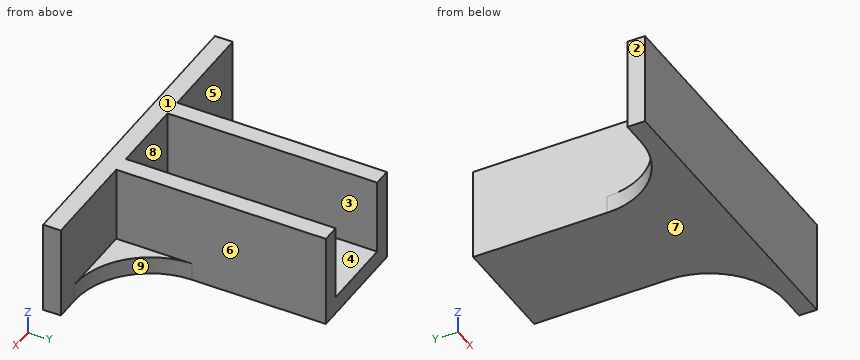
```python
from build123d import *

# Parameters (mm, degrees)
SKETCH1_W           = 22
SKETCH1_H           = 45
BOSS_EXTRUDE1_DEPTH = 18.5
SKETCH2_W           = 15
SKETCH2_H           = 41.5
CUT_EXTRUDE1_DEPTH  = 15
SKETCH3_W           = 20
SKETCH3_H           = 3.5
BOSS_EXTRUDE2_DEPTH = 18.5
BOSS_EXTRUDE3_DEPTH = 3.5


with BuildPart() as part:
    # Sketch1 → Boss-Extrude1 (new body)
    with BuildSketch(Plane.XY):
        with Locations((-5.139289452, 22.368914656)):
            Rectangle(SKETCH1_W, SKETCH1_H)
    extrude(amount=BOSS_EXTRUDE1_DEPTH)

    # Sketch2 → Cut-Extrude1 (cut)
    with BuildSketch(Plane.XY.offset(18.5)):
        with Locations((-5.139289452, 24.118914656)):
            Rectangle(SKETCH2_W, SKETCH2_H)
    extrude(amount=-CUT_EXTRUDE1_DEPTH, mode=Mode.SUBTRACT)

    # Sketch3 → Boss-Extrude2 (add)
    with BuildSketch(Plane(origin=(0, 0, 0), x_dir=(-1, 0, 0), z_dir=(0, 0, -1))):
        with Locations((26.139289452, 1.618914656)):
            Rectangle(SKETCH3_W, SKETCH3_H)
        with Locations((-15.860710548, 1.618914656)):
            Rectangle(SKETCH3_W, SKETCH3_H)
    extrude(amount=-BOSS_EXTRUDE2_DEPTH)

    # Sketch4 → Boss-Extrude3 (add)
    with BuildSketch(Plane(origin=(0, 0, 0), x_dir=(-1, 0, 0), z_dir=(0, 0, -1))):
        with BuildLine():
            Line((31.139289452, 3.368914656), (16.139289452, 3.368914656))
            Line((16.139289452, 3.368914656), (16.139289452, 18.368914656))
            ThreePointArc((16.139289452, 18.368914656), (20.532687735, 7.762312938), (31.139289452, 3.368914656))
        make_face()
        with BuildLine():
            Line((-20.860710548, 3.368914656), (-5.860710548, 3.368914656))
            Line((-5.860710548, 3.368914656), (-5.860710548, 18.368914656))
            ThreePointArc((-5.860710548, 18.368914656), (-10.25410883, 7.762312938), (-20.860710548, 3.368914656))
        make_face()
    extrude(amount=-BOSS_EXTRUDE3_DEPTH)


solid = part.part
```
Source: CAD feature listing. Evaluate the final solid. Frame: model axes, mm. Face numbers are marked on the shaded views. A direction names the side the tool comes from. Round coordinates to 2 decimals unless told otherwise and drop trailing zeros. Loops run counter-clockwise (first coordinate to the right, second up) from the corner with the lowest first, then second, coordinate; pieces in that order, holes last. Notation, with made-up numbers: M -19,33 L -1,33 A15 cw -1,49 Z; hole C -16.5,13.5 d6. An arc over 180 degrees is marked long. Use a Markdown table: item, result. Add a question column.
1. Cut plane C-C, the plane x = -8. Output: boundary loops of the cut face in (y, z).
2. Cut plane A-A, the plane y = 37. Output: boundary loops of the cut face in (x, z), and give its area (3 significant figures).
3. Set-up query: the marked faces 5, 6, 7, 8 and 9. Return all of +Z, -Z, +X, -X, +Y, -Y with unobstructed straight access to the full face (end or side cutting, diameter ignored); none if empty.
4. Pull-direction query (X, two-part tool) for the marked faces 1, 2, 3 and 4; classes: +X half, -X half, draft (parallel to the pull), parting line (faces both ways), or undercut.
5. Contact query for flat-ended pins moving along their axis: pin 1 (2 mm diameter, centred on x = 9.5, z = 3.5, fed in from +Y); pin 2 (4.5 mm diameter, centred on y = 25.5, z = 7.5, fed in from -X); pin 3 (2 mm diameter, centred on x = 16.5, z = 9, fed in from +Y). Output: stop coordinate, or through.
6. Cut plane B-B, the plane z = 6. Output: boundary loops of the cut face in (x, y).
7. Ray query, line 1 along X through (y, z) = (31.5, 17); line 2 along Y through (x, z) = (-25, 12.5); line 3 along Z through (x, y) = (-8, 7). Return the intervals inside material, ascending. Write a range as [from, to].
Solution:
| question | item | result |
|---|---|---|
| 1 | outline | M -0.13,0 L 44.87,0 L 44.87,3.5 L 3.37,3.5 L 3.37,18.5 L -0.13,18.5 Z |
| 2 | outline | M -16.14,0 L 5.86,0 L 5.86,18.5 L 2.36,18.5 L 2.36,3.5 L -12.64,3.5 L -12.64,18.5 L -16.14,18.5 Z |
| 2 | area | 182 mm2 |
| 3 | face 5 | +Z, -X, +Y |
| 3 | face 6 | +Z, +X, +Y |
| 3 | face 7 | -Z, +X, -X, +Y, -Y |
| 3 | face 8 | +Z, +Y |
| 3 | face 9 | +Z, -Z, +X, +Y |
| 4 | face 1 | draft |
| 4 | face 2 | -X half |
| 4 | face 3 | undercut |
| 4 | face 4 | undercut |
| 5 | pin 1 | stops at y = 9.87 |
| 5 | pin 2 | stops at x = -16.14 |
| 5 | pin 3 | stops at y = 3.37 |
| 6 | outline | M -36.14,-0.13 L 25.86,-0.13 L 25.86,3.37 L 5.86,3.37 L 5.86,44.87 L 2.36,44.87 L 2.36,3.37 L -12.64,3.37 L -12.64,44.87 L -16.14,44.87 L -16.14,3.37 L -36.14,3.37 Z |
| 7 | line 1 | x = [-16.14, -12.64], [2.36, 5.86] |
| 7 | line 2 | y = [-0.13, 3.37] |
| 7 | line 3 | z = [0, 3.5] |
